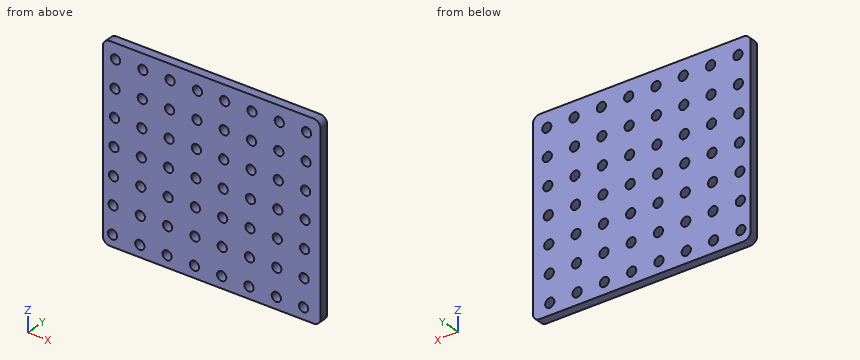
```python
from build123d import *

# Parameters (mm, degrees)
F0_W     = 78.232
F0_H     = 68.43406
F1_DEPTH = 3.175
F3_D     = 3.302
F4_R     = 2.54


with BuildPart() as f1:
    # F0 (on Front) → F1 (new body)
    with BuildSketch(Plane.XZ):
        Rectangle(F0_W, F0_H)
    extrude(amount=F1_DEPTH)

    # F3 (through all)
    with Locations(Plane.XZ.offset(3.175)):
        with Locations((3.775014, -20.257733), (33.008497, -30.060486), (-24.919317, 18.953278), (-6.029386, -20.257733), (33.547649, -0.652228), (-25.817903, -30.060486), (-15.654069, -10.454981), (23.743249, -0.652228), (-5.849669, -10.454981), (-5.669951, -0.652228), (14.478, 28.75603), (4.134449, -0.652228), (-35.622303, -30.060486), (3.954731, -10.454981), (33.727366, 9.150525), (24.102683, 18.953278), (-34.903434, 9.150525), (-35.442586, -20.257733), (-25.638186, -20.257733), (34.0868, 28.75603), (24.2824, 28.75603), (4.6736, 28.75603), (-5.1308, 28.75603), (33.907083, 18.953278), (-5.490234, 9.150525), (13.399697, -30.060486), (-14.9352, 28.75603), (-24.7396, 28.75603), (-35.262869, -10.454981), (-25.458469, -10.454981), (4.314166, 9.150525), (-5.310517, 18.953278), (23.204097, -30.060486), (13.579414, -20.257733), (-35.083151, -0.652228), (4.493883, 18.953278), (-16.013503, -30.060486), (13.759131, -10.454981), (23.383814, -20.257733), (-25.278751, -0.652228), (-15.474351, -0.652228), (14.298283, 18.953278), (33.188214, -20.257733), (-6.209103, -30.060486), (-15.833786, -20.257733), (-34.544, 28.75603), (13.938849, -0.652228), (23.563531, -10.454981), (-25.099034, 9.150525), (-15.294634, 9.150525), (3.595297, -30.060486), (33.367931, -10.454981), (-34.723717, 18.953278), (23.922966, 9.150525), (-15.114917, 18.953278), (14.118566, 9.150525)):
            Hole(F3_D / 2)

    # F4
    f4_edges = [f1.edges().sort_by_distance(p)[0] for p in [
        (-39.116, -1.5875, 34.21703),
        (-39.116, -1.5875, -34.21703),
        (39.116, -1.5875, -34.21703),
        (39.116, -1.5875, 34.21703),
    ]]
    fillet(f4_edges, radius=F4_R)


solid = f1.part
```
For this review, take the finished solid that the model builds, in its own axes (mm). Coordinates: 2 decimals unless noted, no trailing zeros. Answer as a JSON object with one key per item and string values. Group by question number.
1. For probe 1 along Z at (x, y) = (31.5, -0.15), list the stretches that pass through material, from the lowest coordinate up.
2. We need section A-A on y = -1.05. Give the number of separate pieces and of enclosed holes in the cut face, then the cut area to 3 significant figures.
3. Clearance check with a flat-ended pin moving along its axis: P1, Ø1, axis at x = 23.5, z = -10, coming from the +Y side. State where the tip first meets the part, or that it passes through.
Final values:
{
 "1": {"probe 1": "-34.22 to -30.73, -29.39 to 34.22"},
 "2": {"separate pieces": "1", "enclosed holes": "56", "area": "4,870 mm²"},
 "3": {"P1": "through"}
}
